from build123d import *

# Parameters (mm, degrees)
SKETCH1_R           = 57.5
BOSS_EXTRUDE1_DEPTH = 25
SKETCH2_R           = 10
CUT_EXTRUDE1_DEPTH  = 86.073497636
SKETCH3_R           = 3.219002266
CUT_EXTRUDE2_DEPTH  = 17.66963
CIRPATTERN1_START   = 7.330370324
CIRPATTERN1_DEPTH   = 17.669629676


# Read off the part's stored shape, not the designer's step: CirPattern1
with BuildPart() as part:
    # Sketch1 → Boss-Extrude1 (new body)
    with BuildSketch(Plane(origin=(0, 0, 0), x_dir=(1, 0, 0), z_dir=(0, 1, 0))):
        with Locations(Location((0, 0, 0), (0, 0, 270))):
            Circle(SKETCH1_R)
    extrude(amount=BOSS_EXTRUDE1_DEPTH)

    # Sketch2 → Cut-Extrude1 (cut, through all)
    with BuildSketch(Plane(origin=(0, 0, 0), x_dir=(1, 0, 0), z_dir=(0, 1, 0))):
        with Locations(Location((0, 0, 0), (0, 0, 270))):
            Circle(SKETCH2_R)
    extrude(amount=CUT_EXTRUDE1_DEPTH, mode=Mode.SUBTRACT)

    # Sketch3 → Cut-Extrude2 (cut)
    with BuildSketch(Plane(origin=(0, 25, 0), x_dir=(1, 0, 0), z_dir=(0, 1, 0))):
        with Locations((-11.793512299, 0)):
            Circle(SKETCH3_R)
    extrude(amount=-CUT_EXTRUDE2_DEPTH, mode=Mode.SUBTRACT)

    # CirPattern1 outline → CirPattern1 (cut)
    with BuildSketch(Plane(origin=(0, 0, 0), x_dir=(1, 0, 0), z_dir=(0, 1, 0)).offset(CIRPATTERN1_START)):
        with BuildLine():
            ThreePointArc((-5.129596259, -8.584127342), (-7.071067812, -7.071067812), (-8.584127342, -5.129596259))
            ThreePointArc((-8.584127342, -5.129596259), (-10.615450852, -10.615450852), (-5.129596259, -8.584127342))
        make_face()
        with BuildLine():
            ThreePointArc((-5.129596259, 8.584127342), (-10.615450852, 10.615450852), (-8.584127342, 5.129596259))
            ThreePointArc((-8.584127342, 5.129596259), (-7.071067812, 7.071067812), (-5.129596259, 8.584127342))
        make_face()
        with BuildLine():
            ThreePointArc((2.442722354, -9.697066953), (0, -10), (-2.442722354, -9.697066953))
            ThreePointArc((-2.442722354, -9.697066953), (0, -15.012514565), (2.442722354, -9.697066953))
        make_face()
        with BuildLine():
            ThreePointArc((2.442722354, 9.697066953), (0, 15.012514565), (-2.442722354, 9.697066953))
            ThreePointArc((-2.442722354, 9.697066953), (0, 10), (2.442722354, 9.697066953))
        make_face()
        with BuildLine():
            ThreePointArc((8.584127342, -5.129596259), (7.071067812, -7.071067812), (5.129596259, -8.584127342))
            ThreePointArc((5.129596259, -8.584127342), (10.615450852, -10.615450852), (8.584127342, -5.129596259))
        make_face()
        with BuildLine():
            ThreePointArc((8.584127342, 5.129596259), (10.615450852, 10.615450852), (5.129596259, 8.584127342))
            ThreePointArc((5.129596259, 8.584127342), (7.071067812, 7.071067812), (8.584127342, 5.129596259))
        make_face()
        with BuildLine():
            ThreePointArc((9.697066953, 2.442722354), (10, 0), (9.697066953, -2.442722354))
            ThreePointArc((9.697066953, -2.442722354), (15.012514565, 0), (9.697066953, 2.442722354))
        make_face()
    extrude(amount=CIRPATTERN1_DEPTH, mode=Mode.SUBTRACT)


solid = part.part
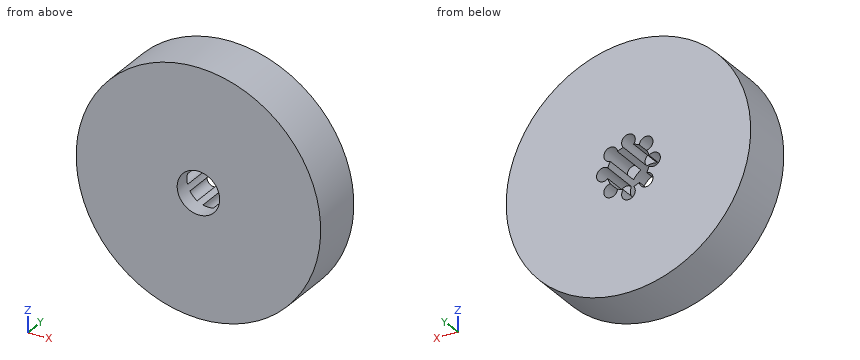
Geometry check sheet. Reference: the model listing, model coordinates, mm. Round coordinates to 2 decimals unless told otherwise and drop trailing zeros. Write each loop counter-clockwise with the first axis right and the second up, starting at its lowest first coordinate (ties: lowest second). Pieces come first, ordered by that corner, then holes.
Item 1: Go/stop test with flat-tipped pins: pin 1 Ø1 at (y, z) = (10.5, -45.5) entering from -X; pin 2 Ø4.5 at (x, z) = (1, -11.5) entering from +Y; pin 3 Ø12 at (x, y) = (-14, 16) entering from -Z; pin 4 Ø2.5 at (x, z) = (-12, 1.5) entering from +Y. Record where each tip stops, or that it passes through.
Determined:
pin 1: stops at x = -35.79
pin 2: stops at y = 25
pin 3: stops at z = -56.94
pin 4: stops at y = 7.33
Item 2: Material ranges on line 1 along X through (y, z) = (18.25, 0); line 2 along Z through (x, y) = (5.5, 14.25); line 3 along Z through (x, y) = (2, 14.5), recorded low to high.
Determined:
line 1: x = -57.5 to -15.01, 15.01 to 57.5
line 2: z = -57.24 to -9.86, 9.86 to 57.24
line 3: z = -57.47 to -14.32, 14.32 to 57.47
Item 3: Section check D-D (x = -34.5). Record the boundary of the cut face in (y, z).
Determined:
outline: (0, -46) - (25, -46) - (25, 46) - (0, 46) - close
Item 4: Section check B-B (z = 0). Record the boundary of the cut face in (x, y).
Determined:
outline: (-57.5, 0) - (-10, 0) - (-10, 7.33) - (-15.01, 7.33) - (-15.01, 25) - (-57.5, 25) - close; (10, 0) - (57.5, 0) - (57.5, 25) - (15.01, 25) - (15.01, 7.33) - (10, 7.33) - close
Item 5: Section check C-C (y = 22.5). Record the boundary of the cut face in (x, z).
Determined:
outline: circle Ø115 at (0, 0); hole (-9.7, -2.44) arc R10 ccw to (-8.58, -5.13) arc R3.22 ccw (long way) to (-5.13, -8.58) arc R10 ccw to (-2.44, -9.7) arc R3.22 ccw (long way) to (2.44, -9.7) arc R10 ccw to (5.13, -8.58) arc R3.22 ccw (long way) to (8.58, -5.13) arc R10 ccw to (9.7, -2.44) arc R3.22 ccw (long way) to (9.7, 2.44) arc R10 ccw to (8.58, 5.13) arc R3.22 ccw (long way) to (5.13, 8.58) arc R10 ccw to (2.44, 9.7) arc R3.22 ccw (long way) to (-2.44, 9.7) arc R10 ccw to (-5.13, 8.58) arc R3.22 ccw (long way) to (-8.58, 5.13) arc R10 ccw to (-9.7, 2.44) arc R3.22 ccw (long way) to start
Item 6: Section check A-A (x = 0). Record the boundary of the cut face in (y, z), plus the area to 3 significant figures.
Determined:
outline: (0, -57.5) - (25, -57.5) - (25, -15.01) - (7.33, -15.01) - (7.33, -10) - (0, -10) - close; (0, 10) - (7.33, 10) - (7.33, 15.01) - (25, 15.01) - (25, 57.5) - (0, 57.5) - close
area: 2,200 mm2
